Source: CAD feature listing. Evaluate the final solid. Frame: model axes, mm. Face numbers are marked on the shaded views. Give positions to 0.01 mm unless a question says otherwise; leave off trailing zeros. Order: outer loops, then holes, each group sorted by start corner. A loop starts at its lowest first (then second) coordinate and runs counter-clockwise, first axis right, second up.
1) Material intervals for line 1 (Y direction, x = 3.25, z = 0.05); line 2 (Z direction, x = 0.25, y = 2.8); line 3 (Y direction, x = 5, z = 0.8), sorted ascending.
2) Section D-D, the plane y = 0.3. Return loops of the section in (x, z).
3) Section C-C, the plane x = -4.5. Return loops of the section in (y, z), plus the area to 3 significant figures.
4) Section B-B, the plane y = 1.4. Return loops of the section in (x, z), plus the area to 3 significant figures.
5) Section A-A, the plane z = 0. Return loops of the section in (x, y), plus the area to 4 significant figures.
6) Draft query along Y for the marked faces 1, 2, 3 and 4. Return one class per face: released by +Y, released by -Y, zero draft, split by the parting line, or undercut.
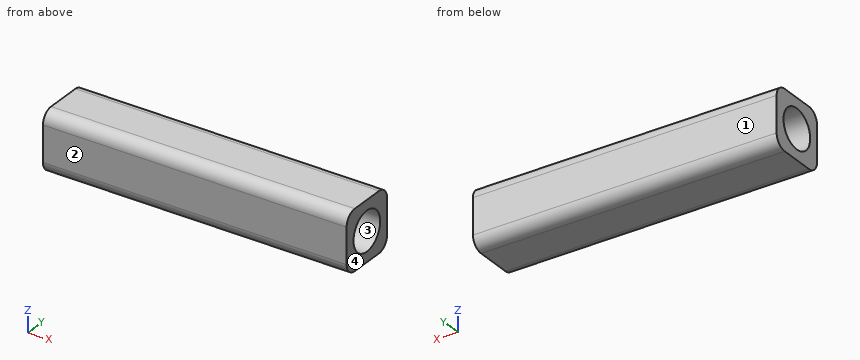
```python
from build123d import *

# Parameters (mm, degrees)
SKETCH1_W               = 25.5
SKETCH1_H               = 5
BOSS_EXTRUDE1_DEPTH     = 5
SKETCH2_R               = 1.65
CUT_EXTRUDE1_DEPTH      = 1
CUT_EXTRUDE1_DEPTH_BACK = 26.5
FILLET1_R               = 1


with BuildPart() as part:
    # Sketch1 → Boss-Extrude1 (new body)
    with BuildSketch(Plane(origin=(0, 0, 0), x_dir=(1, 0, 0), z_dir=(0, 1, 0))):
        Rectangle(SKETCH1_W, SKETCH1_H)
    extrude(amount=BOSS_EXTRUDE1_DEPTH)

    # Sketch2 → Cut-Extrude1 (cut, two sides)
    with BuildSketch(Plane(origin=(12.75, 0, 0), x_dir=(0, 0, -1), z_dir=(1, 0, 0))) as cut_extrude1_sk:
        with Locations((0, 2.5)):
            Circle(SKETCH2_R)
    extrude(amount=CUT_EXTRUDE1_DEPTH, mode=Mode.SUBTRACT)
    extrude(cut_extrude1_sk.sketch, amount=-CUT_EXTRUDE1_DEPTH_BACK, mode=Mode.SUBTRACT)

    # Fillet1
    fillet1_edges = [part.edges().sort_by_distance(p)[0] for p in [
        (0, 5, 2.5),
        (0, 0, 2.5),
        (0, 0, -2.5),
        (0, 5, -2.5),
    ]]
    fillet(fillet1_edges, radius=FILLET1_R)


solid = part.part
```
From the geometry:
1. line 1: y = 0 to 0.85, 4.15 to 5
1. line 2: z = -2.5 to -1.62, 1.62 to 2.5
1. line 3: y = 0 to 1.06, 3.94 to 5
2. outline: (-12.75, -2.21) - (12.75, -2.21) - (12.75, 2.21) - (-12.75, 2.21) - close
3. outline: (0, -1.5) arc R1 ccw to (1, -2.5) - (4, -2.5) arc R1 ccw to (5, -1.5) - (5, 1.5) arc R1 ccw to (4, 2.5) - (1, 2.5) arc R1 ccw to (0, 1.5) - close; hole circle Ø3.3 at (2.5, 0)
3. area: 15.6 mm2
4. outline: (-12.75, -2.5) - (12.75, -2.5) - (12.75, -1.23) - (-12.75, -1.23) - close; (-12.75, 1.23) - (12.75, 1.23) - (12.75, 2.5) - (-12.75, 2.5) - close
4. area: 64.8 mm2
5. outline: (-12.75, 0) - (12.75, 0) - (12.75, 0.85) - (-12.75, 0.85) - close; (-12.75, 4.15) - (12.75, 4.15) - (12.75, 5) - (-12.75, 5) - close
5. area: 43.35 mm2
6. face 1: released by +Y
6. face 2: released by -Y
6. face 3: undercut
6. face 4: zero draft
